Verification items for the finished model (mm, model axes). Give positions to 0.01 mm unless a question says otherwise; leave off trailing zeros. Loops run counter-clockwise (first coordinate to the right, second up) from the corner with the lowest first, then second, coordinate; pieces in that order, holes last. Notation, with made-up numbers: (51.25, 79) - (92.25, 79) arc R24 ccw to (92.25, 98) - close; hole circle Ø6 at (76.5, 55). An arc over 180 degrees is marked (long way). One line per item, written item: value. Start each with the question number.
1. Sectioned sample at A-A (z = 20). Record the cut outline in (x, y) (3 decimals), plus the area to 3 significant figures.
2. Scan lines: L1, parallel to Z at x = 0, y = 2.5; L2, parallel to X at y = 2, z = 20; L3, parallel to Y at x = 3.75, z = 7. Record each from-to range of solid material in increasing order. Write a range as [from, to].
3. Gauge pin test, flat ends, axial feed: pin 1 (1.6 mm diameter, centred on x = 1.5, y = -4, fed in from -Z); pin 2 (3 mm diameter, centred on x = 0, z = 20, fed in from +Y) (3 decimals); pin 3 (5 mm diameter, centred on x = -1.5, z = 55, fed in from -Y). Record the tip position at first contact, or that the pin passes through.
4. Sectioned sample at C-C (z = 54.5). Record the cut outline in (x, y).
5. Sectioned sample at B-B (x = 0). Record the cut outline in (y, z) (3 decimals).
from build123d import *

# Parameters (mm, degrees)
ESQUISSE1_W                     = 10
ESQUISSE1_H                     = 10
BOSS_EXTRU_1_DEPTH              = 150.664880645
ESQUISSE2_W                     = 10
ESQUISSE2_H                     = 2
ENL_V_MAT_EXTRU_1_DEPTH         = 152.079139062
TROU_TARAUD_M3X0_51_D           = 2.5
TROU_TARAUD_M3X0_51_CSINK_D     = 3.05
TROU_TARAUD_M3X0_51_CSINK_ANGLE = 90


with BuildPart() as part:
    # Esquisse1 → Boss.-Extru.1 (new body)
    with BuildSketch(Plane.XY):
        Rectangle(ESQUISSE1_W, ESQUISSE1_H)
    extrude(amount=BOSS_EXTRU_1_DEPTH)

    # Esquisse2 → Enlèv. mat.-Extru.1 (cut, through all)
    with BuildSketch(Plane.ZY.offset(5)):
        with Locations((5, -4)):
            Rectangle(ESQUISSE2_W, ESQUISSE2_H)
        with Locations((57.4, -4)):
            Rectangle(ESQUISSE2_W, ESQUISSE2_H)
    extrude(amount=-ENL_V_MAT_EXTRU_1_DEPTH, mode=Mode.SUBTRACT)

    # Trou taraudé M3x0.51 (through all)
    with Locations(Plane(origin=(0, 5, 0), x_dir=(1, 0, 0), z_dir=(0, 1, 0))):
        with Locations((0, -20)):
            CounterSinkHole(TROU_TARAUD_M3X0_51_D / 2, TROU_TARAUD_M3X0_51_CSINK_D / 2, counter_sink_angle=TROU_TARAUD_M3X0_51_CSINK_ANGLE)


solid = part.part
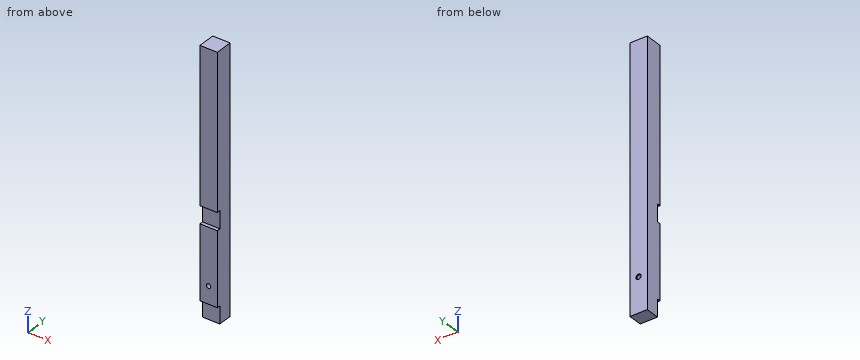
Results are:
1. outline: (-5, -5) - (-1.25, -5) - (-1.25, 4.725) - (-1.525, 5) - (-5, 5) - close; (1.25, -5) - (5, -5) - (5, 5) - (1.525, 5) - (1.25, 4.725) - close
1. area: 74.9 mm^2
2. L1: z = [0, 18.75], [21.25, 150.66]
2. L2: x = [-5, -1.25], [1.25, 5]
2. L3: y = [-3, 5]
3. pin 1: stops at z = 10
3. pin 2: stops at y = 4.975
3. pin 3: stops at y = -3
4. outline: (-5, -3) - (5, -3) - (5, 5) - (-5, 5) - close
5. outline: (-5, 10) - (-3, 10) - (-3, 0) - (5, 0) - (5, 18.475) - (4.725, 18.75) - (-5, 18.75) - close; (-5, 21.25) - (4.725, 21.25) - (5, 21.525) - (5, 150.665) - (-5, 150.665) - (-5, 62.4) - (-3, 62.4) - (-3, 52.4) - (-5, 52.4) - close
